from build123d import *

# Parameters (mm, degrees)
F0_W     = 4
F0_H     = 2.6532998323
F1_DEPTH = 11.5
F0_R     = 3.5
F2_DEPTH = 1
F3_SIZE  = 0.05
F4_SIZE  = 0.05


with BuildPart() as f1:
    # F0 (on Top) → F1 (new body)
    with BuildSketch(Plane.XY):
        with BuildLine():
            Line((-2, 1.3266499161), (2, 1.3266499161))
            ThreePointArc((2, 1.3266499161), (0, 2.4), (-2, 1.3266499161))
        make_face()
        Rectangle(F0_W, F0_H)
        with BuildLine():
            ThreePointArc((-2, -1.3266499161), (0, -2.4), (2, -1.3266499161))
            Line((2, -1.3266499161), (-2, -1.3266499161))
        make_face()
    extrude(amount=F1_DEPTH)

    # F0 (on Top) → F2 (join)
    with BuildSketch(Plane.XY):
        Circle(F0_R)
        with BuildLine():
            ThreePointArc((2, 1.3266499161), (2.2978250586, 0.692820323), (2.4, 0))
            ThreePointArc((2.4, 0), (2.2978250586, -0.692820323), (2, -1.3266499161))
            ThreePointArc((2, -1.3266499161), (0, -2.4), (-2, -1.3266499161))
            ThreePointArc((-2, -1.3266499161), (-2.4, 0), (-2, 1.3266499161))
            ThreePointArc((-2, 1.3266499161), (0, 2.4), (2, 1.3266499161))
        make_face(mode=Mode.SUBTRACT)
        with BuildLine():
            ThreePointArc((2, -1.3266499161), (2.2978250586, -0.692820323), (2.4, 0))
            ThreePointArc((2.4, 0), (2.2978250586, 0.692820323), (2, 1.3266499161))
            Line((2, 1.3266499161), (2, -1.3266499161))
        make_face()
        with BuildLine():
            Line((-2, -1.3266499161), (-2, 1.3266499161))
            ThreePointArc((-2, 1.3266499161), (-2.4, 0), (-2, -1.3266499161))
        make_face()
    extrude(amount=F2_DEPTH)

    # F3
    f3_edges = [f1.edges().sort_by_distance(p)[0] for p in [
        (0, -2.4, 11.5),
        (0, 2.4, 11.5),
    ]]
    chamfer(f3_edges, length=F3_SIZE)

    # F4
    f4_edges = [f1.edges().sort_by_distance(p)[0] for p in [
        (-3.5, 0, 0),
    ]]
    chamfer(f4_edges, length=F4_SIZE)


solid = f1.part
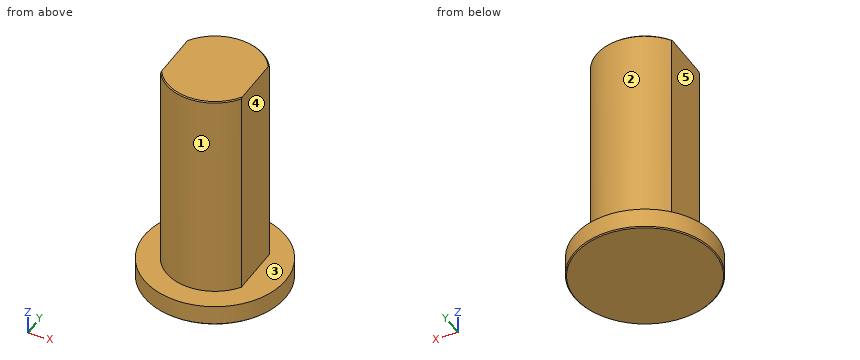
Work out the finished part from the listing and answer in its coordinate system (mm). Face numbers are marked on the shaded views. A direction names the side the tool comes from. Round coordinates to 2 decimals unless told otherwise and drop trailing zeros. Write each loop counter-clockwise with the first axis right and the second up, starting at its lowest first coordinate (ties: lowest second). Pieces come first, ordered by that corner, then holes.
1) A tool of negligible diameter and unlimited length cuts with its end or side. For the marked faces 1, 2, 3, 4 and 5, from which of +Z, -Z, +X, -X, +Y, -Y can it reach the whole face along a straight path? Write none if from no direction.
2) Given pin 1 Ø2 at (y, z) = (0.5, 8.5) entering from +X; pin 2 Ø1.5 at (x, z) = (2, 10) entering from +Y; pin 3 Ø2 at (y, z) = (0, 8.5) entering from -X, each flat-ended and moving along its own axis, determine where each tip first touches the part or whether it passes through.
3) Straight lines are drawn through the part: line 1 (X direction, y = 1.25, z = 10); line 2 (Z direction, x = 0.75, y = -2.5); line 3 (X direction, y = -2, z = 2.25). For each, find the intervals that lie inside material, in ascending order.
4) A cutting plane is placed at A-A (y = 0). Give the vertices of the cut face in (x, z).
5) A cutting plane is placed at B-B (x = 0). Give the vertices of the cut face in (y, z), plus the area to 3 significant figures.
6) A cutting plane is placed at C-C (z = 3). Give the vertices of the cut face in (x, y), plus the area to 3 significant figures.
Completed:
1. face 1: +Z, -Y
1. face 2: +Z, +Y
1. face 3: +Z
1. face 4: +Z, +X, +Y, -Y
1. face 5: +Z, -X, +Y, -Y
2. pin 1: stops at x = 2
2. pin 2: stops at y = 2.05
2. pin 3: stops at x = -2
3. line 1: x = -2 to 2
3. line 2: z = 0 to 1
3. line 3: x = -1.33 to 1.33
4. outline: (-3.5, 0.05) - (-3.45, 0) - (3.45, 0) - (3.5, 0.05) - (3.5, 1) - (2, 1) - (2, 11.5) - (-2, 11.5) - (-2, 1) - (-3.5, 1) - close
5. outline: (-3.5, 0.05) - (-3.45, 0) - (3.45, 0) - (3.5, 0.05) - (3.5, 1) - (2.4, 1) - (2.4, 11.45) - (2.35, 11.5) - (-2.35, 11.5) - (-2.4, 11.45) - (-2.4, 1) - (-3.5, 1) - close
5. area: 57.4 mm2
6. outline: (-2, -1.33) arc R2.4 ccw to (2, -1.33) - (2, 1.33) arc R2.4 ccw to (-2, 1.33) - close
6. area: 16.7 mm2
